Design review of the part shown in the three views and the two pictorial views. Dimensions are in mm from the part's minimum x, y and z. Give positions to 0.01 mm unless a question says otherwise; leave off trailing zeros. Order: outer loops, then holes, each group sorted by start corner. A loop starts at its lowest first (then second) coordinate and runs counter-clockwise, first axis right, second up. Notation, with made-up numbers: (-20, -22) -> (10, -22) arc R24 ccw to (10, -8) -> close; hole circle Ø2 at (36.5, 12). An arc over 180 degrees is marked (long way). Answer in a Markdown table with one row per item. Add a question column.
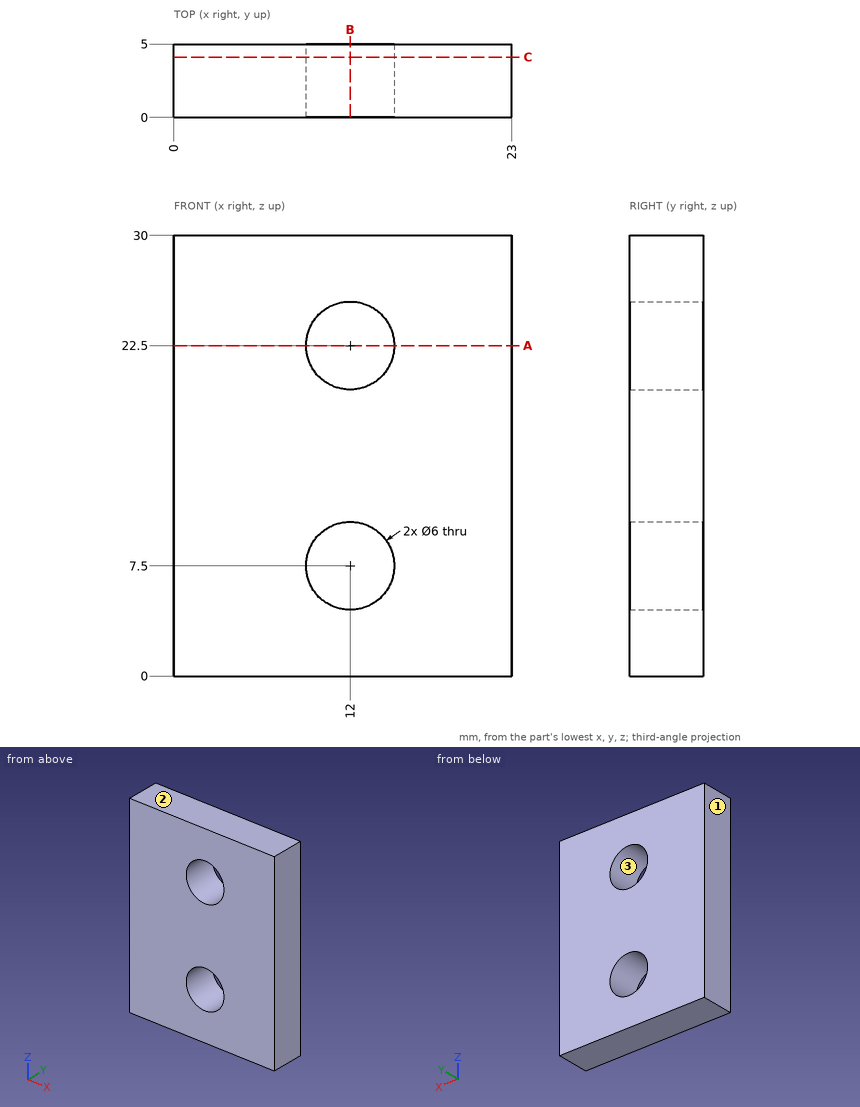
1) Clearance check with a flat-ended pin moving along its axis: P1, Ø10, axis at x = 5.5, z = 10, coming from the -Y side. State where the tip first meets the part, or that it passes through.
2) Add section B-B, the plane x = 12. Write out the cut boundary in (y, z), and give its area (3 significant figures).
3) Add section C-C, the plane y = 4.1. Write out the cut boundary in (x, z).
4) For L1, parallel to Z at x = 12, y = 4.55; L2, parallel to X at y = 1.35, z = 22.5; L3, parallel to Z at x = 9.75, y = 3.2, list the stretches that pass through material, from the lowest coordinate up.
5) Mouldability with a two-part tool opening along X and no side actions: class the marked faces 1, 2 and 3 as +X half, -X half, draft (parallel to the pull), parting line (faces both ways), or undercut.
6) Add section A-A, the plane z = 22.5. Write out the cut boundary in (x, y).
Verdict:
| question | item | result |
|---|---|---|
| 1 | P1 | stops at y = 0 |
| 2 | outline | (0, 0) -> (5, 0) -> (5, 4.5) -> (0, 4.5) -> close; (0, 10.5) -> (5, 10.5) -> (5, 19.5) -> (0, 19.5) -> close; (0, 25.5) -> (5, 25.5) -> (5, 30) -> (0, 30) -> close |
| 2 | area | 90.0 mm2 |
| 3 | outline | (0, 0) -> (23, 0) -> (23, 30) -> (0, 30) -> close; hole circle Ø6 at (12, 7.5); hole circle Ø6 at (12, 22.5) |
| 4 | L1 | z = 0 to 4.5, 10.5 to 19.5, 25.5 to 30 |
| 4 | L2 | x = 0 to 9, 15 to 23 |
| 4 | L3 | z = 0 to 5.52, 9.48 to 20.52, 24.48 to 30 |
| 5 | face 1 | -X half |
| 5 | face 2 | draft |
| 5 | face 3 | undercut |
| 6 | outline | (0, 0) -> (9, 0) -> (9, 5) -> (0, 5) -> close; (15, 0) -> (23, 0) -> (23, 5) -> (15, 5) -> close |
